Job drawing, mm, ordinate dimensions from the low corner. One solid piece. A direction names the side the tool comes from. Give positions to 0.01 mm unless a question says otherwise; leave off trailing zeros. Order: outer loops, then holes, each group sorted by start corner. A loop starts at its lowest first (then second) coordinate and runs counter-clockwise, first axis right, second up. Notation, with made-up numbers: M 82,52 L 102,52 A21 ccw 102,78 Z; hole C -33,9 d4. An arc over 180 degrees is marked long. Put each result on its own line as item: value. Start each with the question number.
1) Cut at A-A (y = 122). Write the cut outline in (x, z).
2) Pin check, flat tips, straight feed: pin 1 (3 mm diameter, centred on x = 36, z = 16.5, fed in from -Y) (3 decimals); pin 2 (4 mm diameter, centred on y = 4, z = 10, fed in from -X); pin 3 (4 mm diameter, centred on x = 108, z = 8.5, fed in from -Y). Stop position of each tip, or through.
3) Cut at B-B (x = 28). Write the cut outline in (y, z) (3 decimals), and give its area (3 significant figures).
4) Cut at C-C (z = 17.5). Write the cut outline in (x, y) (3 decimals), and give its area (3 significant figures).
5) Two-plate mould, pull along X, no slides. Class the marked faces 1, 2, 3 and 4: released by +X, released by -X, zero draft, split by the parting line, or undercut.
6) Tool access for the marked faces 5, 6 and 7: list every direction of +Z, -Z, +X, -X, +Y, -Y with a clear straight run to the whole face (end or side of a thin tool).
7) Drill centre lines: line 1 (Y direction, x = 28, z = 11) (3 decimals); line 2 (X direction, y = 60, z = 12); line 3 (X direction, y = 6, z = 14) (3 decimals). Where is each one in solid material? Low to high. Write a range as [from, to].
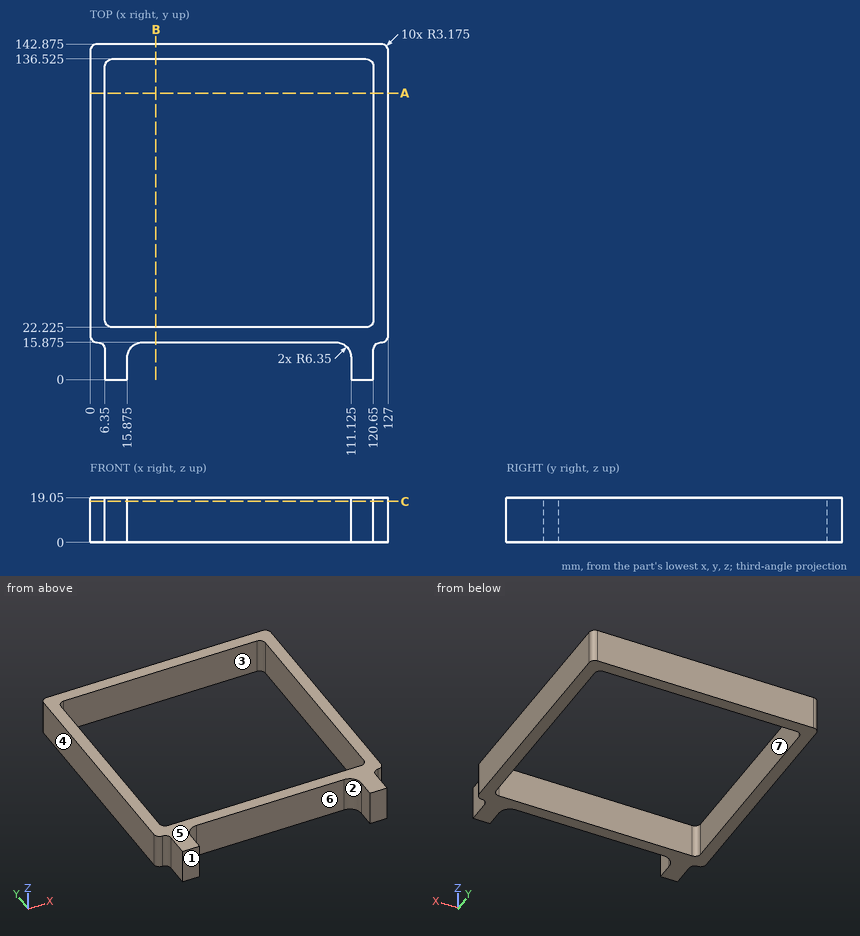
Solution:
1. outline: M 0,0 L 6.35,0 L 6.35,19.05 L 0,19.05 Z; M 120.65,0 L 127,0 L 127,19.05 L 120.65,19.05 Z
2. pin 1: y = 15.875
2. pin 2: x = 6.35
2. pin 3: y = 13.13
3. outline: M 15.875,0 L 22.225,0 L 22.225,19.05 L 15.875,19.05 Z; M 136.525,0 L 142.875,0 L 142.875,19.05 L 136.525,19.05 Z
3. area: 242 mm²
4. outline: M 0,19.05 A3.175 ccw 3.175,15.875 A3.175 cw 6.35,12.7 L 6.35,0 L 15.875,0 L 15.875,9.525 A6.35 cw 22.225,15.875 L 104.775,15.875 A6.35 cw 111.125,9.525 L 111.125,0 L 120.65,0 L 120.65,12.7 A3.175 cw 123.825,15.875 A3.175 ccw 127,19.05 L 127,139.7 A3.175 ccw 123.825,142.875 L 3.175,142.875 A3.175 ccw 0,139.7 Z; hole M 6.35,25.4 A3.175 ccw 9.525,22.225 L 117.475,22.225 A3.175 ccw 120.65,25.4 L 120.65,133.35 A3.175 ccw 117.475,136.525 L 9.525,136.525 A3.175 ccw 6.35,133.35 Z
4. area: 3,390 mm²
5. face 1: zero draft
5. face 2: undercut
5. face 3: undercut
5. face 4: released by -X
6. face 5: +Z, +X, -X, +Y, -Y
6. face 6: +Z, -Z, -Y
6. face 7: +Z, -Z
7. line 1: [15.875, 22.225], [136.525, 142.875]
7. line 2: [0, 6.35], [120.65, 127]
7. line 3: [6.35, 15.875], [111.125, 120.65]
